Read the model definition and answer for the solid it produces. Units are mm, in the model's axes. A direction names the side the tool comes from. Give positions to 0.01 mm unless a question says otherwise; leave off trailing zeros. Loops run counter-clockwise (first coordinate to the right, second up) from the corner with the lowest first, then second, coordinate; pieces in that order, holes last. Notation, with made-up numbers: (79, 1.5) -> (86, 1.5) arc R33 cw to (86, 29.5) -> close; hole circle Ø8 at (68.25, 66.5). An arc over 180 degrees is marked (long way). Write each question's results on one line, items separated by ' | '. Start each with the question number.
Item 1: Section A-A on y = 6 is taken. Write down the section's boundary in (x, z).
Item 2: Section B-B on z = 5 is taken. Write down the section's boundary in (x, y), and give its area (3 significant figures).
Item 3: Section C-C on x = 5 is taken. Write down the section's boundary in (y, z), and give its area (3 significant figures).
Item 4: Which of the six approach directions +Z, -Z, +X, -X, +Y, -Y give full straight-line access (tool end or side, diameter ignored) to faces 1 (the flat face through (0, 11, 3)), 2 (the cylindrical face through (8.39, 8.58, -5.12)), 3 (the flat face through (10.392, 1, 11))?
Item 5: Determine the mould class of faces 4 (the flat face through (11, 0, -5)), 5 (the flat face through (0, 11, -2)), 6 (the flat face through (10.392, 1, 6)) for opening direction X: +X half, -X half, draft (parallel to the pull), parting line (faces both ways), or undercut.
Item 6: Each of these flat-tipped pins is pushed along its axis until it touches: P1, Ø6, axis at y = 9, z = -1, coming from the +X side; P2, Ø1.5, axis at y = 7, z = 3, coming from the +X side; P3, Ø8, axis at x = -10, z = 3.5, coming from the -Y side; P4, Ø12, axis at x = -10.5, z = -4, coming from the -Y side. Where does it stop, or does it pass through?
Item 7: Find the intervals of material crossed by line 1 (Z direction, x = 10, y = 4); line 2 (Y direction, x = -6.25, z = -8.25); line 3 (X direction, y = 8.75, z = 2), in increasing order.
Item 8: Section D-D on y = 2 is taken. Write down the section's boundary in (x, z).
```python
from build123d import *

# Parameters (mm, degrees)
SKETCH1_W           = 35
SKETCH1_H           = 23.5
BOSS_EXTRUDE1_DEPTH = 12
CUT_EXTRUDE1_DEPTH  = 32.662280398
CUT_EXTRUDE2_DEPTH  = 32.662280398
SKETCH5_W           = 26.392304845
SKETCH5_H           = 23.5
CUT_EXTRUDE3_DEPTH  = 12
SKETCH6_W           = 14.786732963
SKETCH6_H           = 2.5
CUT_EXTRUDE4_DEPTH  = 25.255154091


with BuildPart() as part:
    # Sketch1 → Boss-Extrude1 (new body)
    with BuildSketch(Plane(origin=(0, 0, 0), x_dir=(1, 0, 0), z_dir=(0, 1, 0))):
        Rectangle(SKETCH1_W, SKETCH1_H)
    extrude(amount=BOSS_EXTRUDE1_DEPTH)

    # Sketch3 → Cut-Extrude1 (cut, through all)
    with BuildSketch(Plane.XY.offset(11.75)):
        with BuildLine():
            Line((17.5, 12), (0, 12))
            ThreePointArc((0, 12), (8.485281374, 8.485281374), (12, 0))
            Line((12, 0), (17.5, 0))
            Line((17.5, 0), (17.5, 12))
        make_face()
    extrude(amount=-CUT_EXTRUDE1_DEPTH, mode=Mode.SUBTRACT)

    # Sketch4 → Cut-Extrude2 (cut, through all)
    with BuildSketch(Plane.XY.offset(11.75)):
        with BuildLine():
            Line((-16, 1.5), (10.392304845, 1.5))
            ThreePointArc((10.392304845, 1.5), (6.873863542, 7.937253933), (0, 10.5))
            Line((0, 10.5), (-16, 10.5))
            Line((-16, 10.5), (-16, 1.5))
        make_face()
    extrude(amount=-CUT_EXTRUDE2_DEPTH, mode=Mode.SUBTRACT)

    # Sketch5 → Cut-Extrude3 (cut)
    with BuildSketch(Plane(origin=(0, 1.5, 0), x_dir=(1, 0, 0), z_dir=(0, 1, 0))):
        with Locations((-2.803847578, 0)):
            Rectangle(SKETCH5_W, SKETCH5_H)
    extrude(amount=-CUT_EXTRUDE3_DEPTH, mode=Mode.SUBTRACT)

    # Sketch6 → Cut-Extrude4 (cut, through all)
    with BuildSketch(Plane(origin=(0, 12, 0), x_dir=(1, 0, 0), z_dir=(0, 1, 0))):
        with Locations((7.393366482, -8.60416966)):
            Rectangle(SKETCH6_W, SKETCH6_H)
        with Locations((7.393366482, -3.10416966)):
            Rectangle(SKETCH6_W, SKETCH6_H)
        with Locations((7.393366482, 2.39583034)):
            Rectangle(SKETCH6_W, SKETCH6_H)
        with Locations((7.393366482, 7.89583034)):
            Rectangle(SKETCH6_W, SKETCH6_H)
    extrude(amount=-CUT_EXTRUDE4_DEPTH, mode=Mode.SUBTRACT)


solid = part.part
```
Findings:
1) outline: (-17.5, -11.75) -> (-16, -11.75) -> (-16, 11.75) -> (-17.5, 11.75) -> close; (8.62, -11.75) -> (10.39, -11.75) -> (10.39, -9.15) -> (8.62, -9.15) -> close; (8.62, -6.65) -> (10.39, -6.65) -> (10.39, -3.65) -> (8.62, -3.65) -> close; (8.62, -1.15) -> (10.39, -1.15) -> (10.39, 1.85) -> (8.62, 1.85) -> close; (8.62, 4.35) -> (10.39, 4.35) -> (10.39, 7.35) -> (8.62, 7.35) -> close; (8.62, 9.85) -> (10.39, 9.85) -> (10.39, 11.75) -> (8.62, 11.75) -> close
2) outline: (-17.5, 0) -> (-16, 0) -> (-16, 10.5) -> (0, 10.5) arc R10.5 cw to (10.39, 1.5) -> (10.39, 0) -> (12, 0) arc R12 ccw to (0, 12) -> (-17.5, 12) -> close | area: 68.6 mm2
3) outline: (9.23, -11.75) -> (10.91, -11.75) -> (10.91, -9.15) -> (9.23, -9.15) -> close; (9.23, -6.65) -> (10.91, -6.65) -> (10.91, -3.65) -> (9.23, -3.65) -> close; (9.23, -1.15) -> (10.91, -1.15) -> (10.91, 1.85) -> (9.23, 1.85) -> close; (9.23, 4.35) -> (10.91, 4.35) -> (10.91, 7.35) -> (9.23, 7.35) -> close; (9.23, 9.85) -> (10.91, 9.85) -> (10.91, 11.75) -> (9.23, 11.75) -> close | area: 22.6 mm2
4) face 1: +X, +Y, -Y | face 2: +Z, -Z, +X, +Y | face 3: +Z, -Z, -Y
5) face 4: draft | face 5: +X half | face 6: undercut
6) P1: x = 10.39 | P2: x = -16 | P3: y = 10.5 | P4: y = 0
7) line 1: -11.75 to -9.15, -6.65 to -3.65, -1.15 to 1.85, 4.35 to 7.35, 9.85 to 11.75 | line 2: 10.5 to 12 | line 3: -17.5 to -16
8) outline: (-17.5, -11.75) -> (-16, -11.75) -> (-16, 11.75) -> (-17.5, 11.75) -> close; (10.31, -11.75) -> (11.83, -11.75) -> (11.83, -9.15) -> (10.31, -9.15) -> close; (10.31, -6.65) -> (11.83, -6.65) -> (11.83, -3.65) -> (10.31, -3.65) -> close; (10.31, -1.15) -> (11.83, -1.15) -> (11.83, 1.85) -> (10.31, 1.85) -> close; (10.31, 4.35) -> (11.83, 4.35) -> (11.83, 7.35) -> (10.31, 7.35) -> close; (10.31, 9.85) -> (11.83, 9.85) -> (11.83, 11.75) -> (10.31, 11.75) -> close
